from build123d import *

# Parameters (mm, degrees)
SKETCH_3_R          = 3.4
EXTRUDE_1_DEPTH     = 2421
CUT_EXTRUDE_3_DEPTH = 3297


with BuildPart() as part:
    # 草图3 → 凸台-拉伸1 (new body)
    with BuildSketch(Plane(origin=(0, 0, 0), x_dir=(0, 0, -1), z_dir=(1, 0, 0))):
        with BuildLine():
            Line((-15.5, -20), (-4.5, -20))
            Line((-4.5, -20), (-4.5, -19.5))
            Line((-4.5, -19.5), (-4.1, -19.5))
            Line((-4.1, -19.5), (-4.1, -16.2))
            Line((-4.1, -16.2), (-6.4, -16.2))
            Line((-6.4, -16.2), (-6.4, -18.2))
            Line((-6.4, -18.2), (-10.25, -18.2))
            Line((-10.25, -18.2), (-10.25, -11.522792206))
            Line((-10.25, -11.522792206), (-5.479130441, -6.751922647))
            Line((-5.479130441, -6.751922647), (5.479130441, -6.751922647))
            Line((5.479130441, -6.751922647), (10.25, -11.522792206))
            Line((10.25, -11.522792206), (10.25, -18.2))
            Line((10.25, -18.2), (6.4, -18.2))
            Line((6.4, -18.2), (6.4, -16.2))
            Line((6.4, -16.2), (4.1, -16.2))
            Line((4.1, -16.2), (4.1, -19.5))
            Line((4.1, -19.5), (4.5, -19.5))
            Line((4.5, -19.5), (4.5, -20))
            Line((4.5, -20), (15.5, -20))
            ThreePointArc((15.5, -20), (18.681980515, -18.681980515), (20, -15.5))
            Line((20, -15.5), (20, -4.5))
            Line((20, -4.5), (19.5, -4.5))
            Line((19.5, -4.5), (19.5, -4.1))
            Line((19.5, -4.1), (16.2, -4.1))
            Line((16.2, -4.1), (16.2, -6.4))
            Line((16.2, -6.4), (18.2, -6.4))
            Line((18.2, -6.4), (18.2, -10.25))
            Line((18.2, -10.25), (11.522792206, -10.25))
            Line((11.522792206, -10.25), (6.751922647, -5.479130441))
            Line((6.751922647, -5.479130441), (6.751922647, 5.479130441))
            Line((6.751922647, 5.479130441), (11.522792206, 10.25))
            Line((11.522792206, 10.25), (18.2, 10.25))
            Line((18.2, 10.25), (18.2, 6.4))
            Line((18.2, 6.4), (16.2, 6.4))
            Line((16.2, 6.4), (16.2, 4.1))
            Line((16.2, 4.1), (19.5, 4.1))
            Line((19.5, 4.1), (19.5, 4.5))
            Line((19.5, 4.5), (20, 4.5))
            Line((20, 4.5), (20, 15.5))
            ThreePointArc((20, 15.5), (18.681980515, 18.681980515), (15.5, 20))
            Line((15.5, 20), (4.5, 20))
            Line((4.5, 20), (4.5, 19.5))
            Line((4.5, 19.5), (4.1, 19.5))
            Line((4.1, 19.5), (4.1, 16.2))
            Line((4.1, 16.2), (6.4, 16.2))
            Line((6.4, 16.2), (6.4, 18.2))
            Line((6.4, 18.2), (10.25, 18.2))
            Line((10.25, 18.2), (10.25, 11.522792206))
            Line((10.25, 11.522792206), (5.479130441, 6.751922647))
            Line((5.479130441, 6.751922647), (-5.479130441, 6.751922647))
            Line((-5.479130441, 6.751922647), (-10.25, 11.522792206))
            Line((-10.25, 11.522792206), (-10.25, 18.2))
            Line((-10.25, 18.2), (-6.4, 18.2))
            Line((-6.4, 18.2), (-6.4, 16.2))
            Line((-6.4, 16.2), (-4.1, 16.2))
            Line((-4.1, 16.2), (-4.1, 19.5))
            Line((-4.1, 19.5), (-4.5, 19.5))
            Line((-4.5, 19.5), (-4.5, 20))
            Line((-4.5, 20), (-15.5, 20))
            ThreePointArc((-15.5, 20), (-18.681980515, 18.681980515), (-20, 15.5))
            Line((-20, 15.5), (-20, 4.5))
            Line((-20, 4.5), (-19.5, 4.5))
            Line((-19.5, 4.5), (-19.5, 4.1))
            Line((-19.5, 4.1), (-16.2, 4.1))
            Line((-16.2, 4.1), (-16.2, 6.4))
            Line((-16.2, 6.4), (-18.2, 6.4))
            Line((-18.2, 6.4), (-18.2, 10.25))
            Line((-18.2, 10.25), (-11.522792206, 10.25))
            Line((-11.522792206, 10.25), (-6.751922647, 5.479130441))
            Line((-6.751922647, 5.479130441), (-6.751922647, -5.479130441))
            Line((-6.751922647, -5.479130441), (-11.522792206, -10.25))
            Line((-11.522792206, -10.25), (-18.2, -10.25))
            Line((-18.2, -10.25), (-18.2, -6.4))
            Line((-18.2, -6.4), (-16.2, -6.4))
            Line((-16.2, -6.4), (-16.2, -4.1))
            Line((-16.2, -4.1), (-19.5, -4.1))
            Line((-19.5, -4.1), (-19.5, -4.5))
            Line((-19.5, -4.5), (-20, -4.5))
            Line((-20, -4.5), (-20, -15.5))
            ThreePointArc((-20, -15.5), (-18.681980515, -18.681980515), (-15.5, -20))
        make_face()
        Circle(SKETCH_3_R, mode=Mode.SUBTRACT)
    extrude(amount=EXTRUDE_1_DEPTH)

    # 草图4 → 切除-拉伸3 (cut)
    with BuildSketch(Plane(origin=(2421, -20, 15.5), x_dir=(0, 0, 1), z_dir=(-1, 0, 0))):
        with BuildLine():
            Line((-3.75, 31.75), (3, 31.75))
            Line((3, 31.75), (3, 35.5))
            ThreePointArc((3, 35.5), (2.121320344, 37.621320344), (0, 38.5))
            Line((0, 38.5), (-3.75, 38.5))
            Line((-3.75, 38.5), (-3.75, 31.75))
        make_face()
        with BuildLine():
            Line((-3.75, 8.25), (-3.75, 1.5))
            Line((-3.75, 1.5), (0, 1.5))
            ThreePointArc((0, 1.5), (2.121320344, 2.378679656), (3, 4.5))
            Line((3, 4.5), (3, 8.25))
            Line((3, 8.25), (-3.75, 8.25))
        make_face()
        with BuildLine():
            Line((-27.25, 8.25), (-34, 8.25))
            Line((-34, 8.25), (-34, 4.5))
            ThreePointArc((-34, 4.5), (-33.121320344, 2.378679656), (-31, 1.5))
            Line((-31, 1.5), (-27.25, 1.5))
            Line((-27.25, 1.5), (-27.25, 8.25))
        make_face()
        with BuildLine():
            Line((-27.25, 31.75), (-27.25, 38.5))
            Line((-27.25, 38.5), (-31, 38.5))
            ThreePointArc((-31, 38.5), (-33.121320344, 37.621320344), (-34, 35.5))
            Line((-34, 35.5), (-34, 31.75))
            Line((-34, 31.75), (-27.25, 31.75))
        make_face()
    extrude(amount=CUT_EXTRUDE_3_DEPTH, mode=Mode.SUBTRACT)


solid = part.part
Can you work these out from the model? Positions are in its coordinate system, mm. Coordinates: 2 decimals unless noted, no trailing zeros. Use one line per item in the form item = value.
Q1. For P1, Ø3.5, axis at x = 1172, z = 17.5, coming from the +Y side; P2, Ø2, axis at x = 1437.5, y = -17, coming from the -Z side; P3, Ø1.7, axis at x = 1616, z = -17.5, coming from the -Y side, each with a flat end and sliding along its axis, tell me the tip position at first contact or that it passes through.
Model answer:
P1 = 19.99
P2 = -19.97
P3 = -19.85
Q2. If we section it at A-A (x = 584.5): State how many separate pieces and enclosed holes the cut face has, then the cut area to 3 significant figures.
Model answer:
separate_pieces = 1
enclosed_holes = 5
area = 500 mm^2
Q3. I need wall thicknesses on line 1 along Y through (x, z) = (1582, 5); line 2 along Y through (x, z) = (666, 12); line 3 along Z through (x, y) = (459.5, 17). Which ranges of each line are inside material? Lowest first, please. Write a range as from..to.
Model answer:
line_1 = -20..-16.2, -6.75..6.75, 16.2..20
line_2 = -20..-18.5, -11.75..-10.25, 10.25..11.75, 18.5..20
line_3 = -19.74..-18.1, -11.75..-10.25, -6.4..-4.1, 4.1..6.4, 10.25..11.75, 18.1..19.74
